For this review, use the dimensioned drawing (mm, ordinates from the lowest corner) and the shaded views. A direction names the side the tool comes from. Give positions to 0.01 mm unless a question says otherwise; leave off trailing zeros. Write each loop counter-clockwise with the first axis right and the second up, starting at its lowest first coordinate (ties: lowest second). Pieces come first, ordered by that corner, then holes. Notation, with made-up numbers: M 62.5,-19.75 L 89.5,-19.75 A22 ccw 89.5,15.25 Z; hole C 84.5,20 d10. An arc over 180 degrees is marked long. Use a Markdown table: item, result. Add a question column.
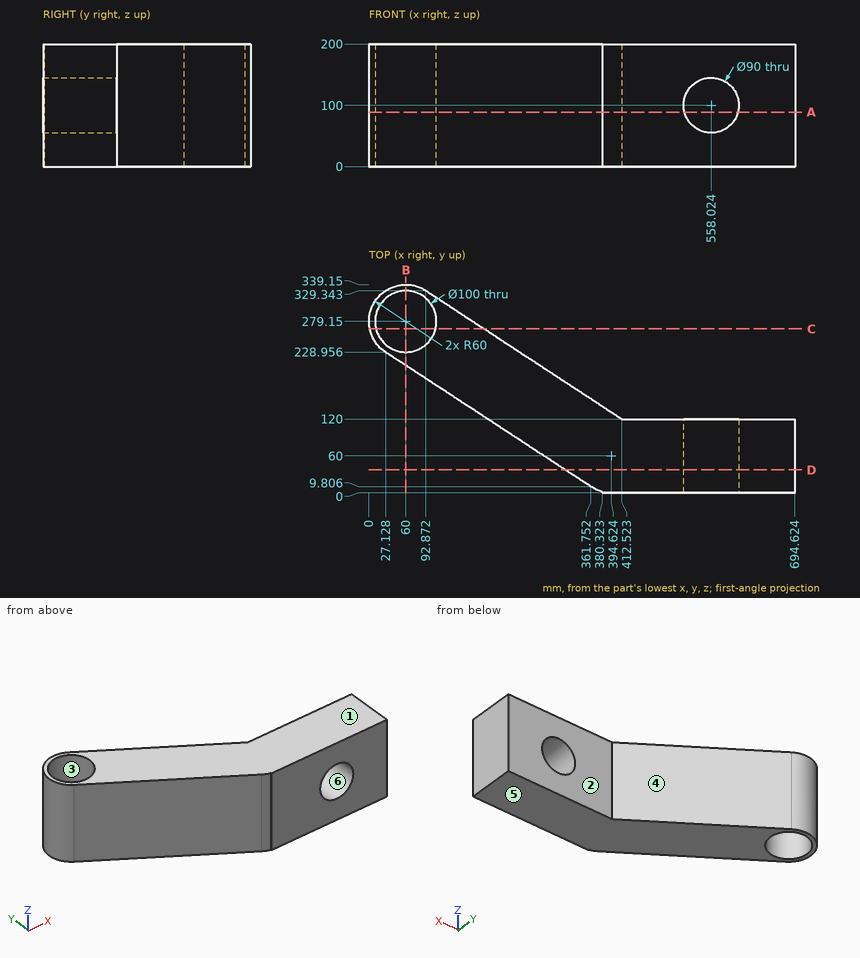
(1) For pin 1 (2 mm diameter, centred on y = 138.5, z = 74, fed in from +X); pin 2 (12 mm diameter, centred on y = 294, z = 35, fed in from +X); pin 3 (3 mm diameter, centred on x = 335, z = 37, fed in from +Y), all flat-tipped, find the tip position at first contact; note any pin that passes through.
(2) Add section D-D on y = 37. Give the boundary of the cut face in (x, z) (1 decimal).
(3) The part is to be moulded in two halves that separate along X. For the marked faces 3, 4, 5 and 6, say which applies: released by +X, released by -X, zero draft, split by the parting line, or undercut.
(4) Add section A-A on z = 89. Give the number of separate pieces and of enclosed holes in the cut face, then the cut area to 3 significant figures.
(5) Add section C-C on y = 267. Give the boundary of the cut face in (x, z) (1 decimal).
(6) Machinability: for the marked faces 1 and 2, which of the approach directions +Z, -Z, +X, -X, +Y, -Y give a long, thin tool a straight path to every point of the face, cutting with its end or side? Answer none if there is none.
(7) Wall thickness on L1, parallel to Y at x = 60, z = 52; L2, parallel to Y at x = 428, z = 189; L3, parallel to X at y = 302, z = 86 (1 decimal): over which ranges is each line inside the solid? List them lowest first.
(8) Add section B-B on x = 60. Give the boundary of the cut face in (y, z).
From the geometry:
| question | item | result |
|---|---|---|
| 1 | pin 1 | stops at x = 385.8 |
| 1 | pin 2 | stops at x = 156 |
| 1 | pin 3 | stops at y = 171.75 |
| 2 | outline | M 320.2,0 L 694.6,0 L 694.6,200 L 320.2,200 Z; hole C 558,100 d90 |
| 3 | face 3 | undercut |
| 3 | face 4 | released by +X |
| 3 | face 5 | zero draft |
| 3 | face 6 | undercut |
| 4 | separate pieces | 2 |
| 4 | enclosed holes | 1 |
| 4 | area | 71,300 mm^2 |
| 5 | outline | M 1.2,0 L 11.5,0 L 11.5,200 L 1.2,200 Z; M 108.5,0 L 188.1,0 L 188.1,200 L 108.5,200 Z |
| 6 | face 1 | +Z, +X, -X, +Y, -Y |
| 6 | face 2 | +Z, -Z, +X, +Y |
| 7 | L1 | y = 207.43 to 229.15, 329.15 to 339.15 |
| 7 | L2 | y = 0 to 120 |
| 7 | L3 | x = 4.5 to 15.5, 104.5 to 134.6 |
| 8 | outline | M 207.43,0 L 229.15,0 L 229.15,200 L 207.43,200 Z; M 329.15,0 L 339.15,0 L 339.15,200 L 329.15,200 Z |
